```python
from build123d import *

# Parameters (mm, degrees)
BOSS_EXTRUDE1_DEPTH      = 10
BOSS_EXTRUDE1_DEPTH_BACK = 10
SKETCH4_R                = 2.25
CUT_EXTRUDE1_DEPTH       = 16


with BuildPart() as part:
    # Sketch2 → Revolve1 (revolve)
    with BuildSketch(Plane.XY):
        Polygon((-42.039607805, -2), (-42.039607805, 0), (-43.951704155, 0), (-43.951704155, -4), (-34.016778293, -4), (0, -4), (0, 0), (-40, 0), (-40, -2), align=None)
    revolve(axis=Axis((0, 100, 0), (0, -1, 0)))

    # Sketch3 → Boss-Extrude1 (add, two sides)
    with BuildSketch(Plane.XY) as boss_extrude1_sk:
        with BuildLine():
            add(Edge.make_bspline(
                [(5, -4), (-2.972410052, -4), (-7.432745191, -9)],
                knots=[1.570796327, 1.570796327, 1.570796327, 2.547844784, 2.547844784, 2.547844784], degree=2, weights=[1, 0.883026434, 1]))
            Line((5, -4), (-35, -4))
            Line((-35, -4), (-35, -9))
            Line((-35, -9), (-7.432745191, -9))
        make_face()
    extrude(amount=BOSS_EXTRUDE1_DEPTH)
    extrude(boss_extrude1_sk.sketch, amount=-BOSS_EXTRUDE1_DEPTH_BACK)

    # Sketch4 → Cut-Extrude1 (cut)
    with BuildSketch(Plane.XZ.offset(9)):
        with Locations((-30, 0)):
            Circle(SKETCH4_R)
        with Locations((-15, 0)):
            Circle(SKETCH4_R)
    extrude(amount=-CUT_EXTRUDE1_DEPTH, mode=Mode.SUBTRACT)


solid = part.part
```
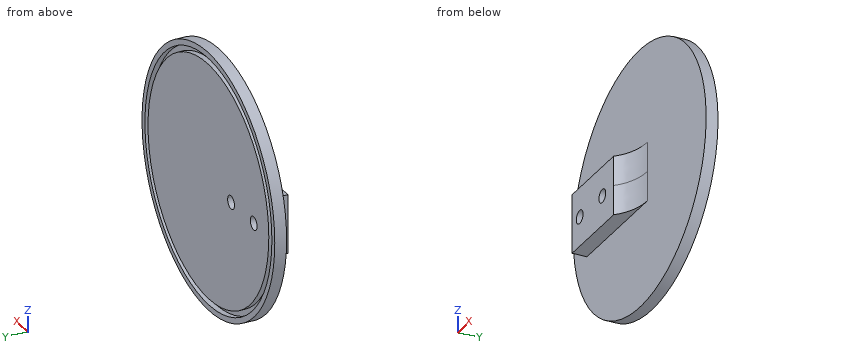
Geometry: final body of the model. Coordinates: model frame, mm. Round coordinates to 2 decimals unless told otherwise and drop trailing zeros. Order: outer loops, then holes, each group sorted by start corner. A loop starts at its lowest first (then second) coordinate and runs counter-clockwise, first axis right, second up. Notation, with made-up numbers: M -24.75,57 L 10.25,57 A24 ccw 10.25,95 Z; hole C 37,-5.75 d7. An arc over 180 degrees is marked long. Use one line per item in the form item = value. Start each with the question number.
Q1. Material intervals for line 1 (Z direction, x = 0, y = -1.2); line 2 (Z direction, x = -15, y = -6.5); line 3 (Z direction, x = 29.5, y = -0.25), sorted ascending. Write a range as [from, to].
Q2. Pin query (flat end, axial travel): pin 1 Ø5 at (x, y) = (-1, -1.5) entering from -Z; pin 2 Ø4 at (x, z) = (-1, -19.5) entering from +Y; pin 3 Ø10 at (x, z) = (6.5, -4.5) entering from -Y; pin 4 Ø3.5 at (x, z) = (-30, 0) entering from +Y. Return the tip coordinate at first contact, or that it passes through.
Q3. Cut plane D-D (y = -7.25). Count the separate pieces of the cut face and the enclosed holes in it, and give its area (3 significant figures).
Q4. Cut plane A-A (x = -30). Return loops of the section in (y, z).
Q5. Cut plane B-B (z = 13). Return loops of the section in (x, y).
Q6. Cut plane C-C (x = -15). Return loops of the section in (y, z), and give its area (3 significant figures).
Geometry results:
q1.line_1 = [-43.95, -42.04], [-40, 40], [42.04, 43.95]
q1.line_2 = [-10, -2.25], [2.25, 10]
q1.line_3 = [-32.58, -29.95], [-27.01, 27.01], [29.95, 32.58]
q2.pin_1 = -43.95
q2.pin_2 = 0
q2.pin_3 = -4.31
q2.pin_4 = through
q3.separate_pieces = 1
q3.enclosed_holes = 2
q3.area = 558 mm^2
q4.outline = M -9,-10 L -4,-10 L -4,-32.12 L 0,-32.12 L 0,-29.45 L -2,-29.45 L -2,-26.46 L 0,-26.46 L 0,-2.25 L -9,-2.25 Z; M -9,2.25 L 0,2.25 L 0,26.46 L -2,26.46 L -2,29.45 L 0,29.45 L 0,32.12 L -4,32.12 L -4,10 L -9,10 Z
q5.outline = M -41.99,-4 L 41.99,-4 L 41.99,0 L 39.98,0 L 39.98,-2 L 37.83,-2 L 37.83,0 L -37.83,0 L -37.83,-2 L -39.98,-2 L -39.98,0 L -41.99,0 Z
q6.outline = M -9,-10 L -4,-10 L -4,-41.31 L 0,-41.31 L 0,-39.27 L -2,-39.27 L -2,-37.08 L 0,-37.08 L 0,-2.25 L -9,-2.25 Z; M -9,2.25 L 0,2.25 L 0,37.08 L -2,37.08 L -2,39.27 L 0,39.27 L 0,41.31 L -4,41.31 L -4,10 L -9,10 Z
q6.area = 381 mm^2
